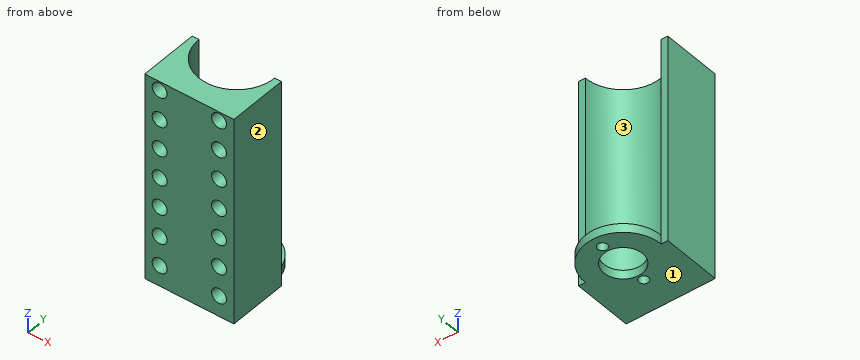
```python
from build123d import *

# Parameters (mm, degrees)
SKETCH1_R                = 12.75
SKETCH1_R_2              = 6.5
BOSS_EXTRUDE1_DEPTH      = 3
BOSS_EXTRUDE2_DEPTH      = 67
BOSS_EXTRUDE2_DEPTH_BACK = 3
SKETCH4_R                = 2.515
CUT_EXTRUDE1_DEPTH       = 6
LPATTERN1_COUNT          = 2
LPATTERN1_PITCH          = 20
LPATTERN1_COUNT_DIR2     = 7
LPATTERN1_PITCH_DIR2     = 10
SKETCH5_R                = 1.65
CUT_EXTRUDE2_DEPTH       = 75


with BuildPart() as part:
    # Sketch1 → Boss-Extrude1 (new body)
    with BuildSketch(Plane.XY):
        Circle(SKETCH1_R)
        Circle(SKETCH1_R_2, mode=Mode.SUBTRACT)
    extrude(amount=BOSS_EXTRUDE1_DEPTH)

    # Sketch2 → Boss-Extrude2 (add, two sides)
    with BuildSketch(Plane.XY.offset(3)) as boss_extrude2_sk:
        with BuildLine():
            Line((15, -20), (15, 0))
            Line((15, 0), (12.75, 0))
            ThreePointArc((12.75, 0), (0, -12.75), (-12.75, 0))
            Line((-12.75, 0), (-15, 0))
            Line((-15, 0), (-15, -20))
            Line((-15, -20), (15, -20))
        make_face()
    extrude(amount=BOSS_EXTRUDE2_DEPTH)
    extrude(boss_extrude2_sk.sketch, amount=-BOSS_EXTRUDE2_DEPTH_BACK)

    # Sketch4 → Cut-Extrude1 (cut)
    with BuildSketch(Plane.XZ.offset(20)):
        with Locations((-10, 67)):
            Circle(SKETCH4_R)
    cut_extrude1 = extrude(amount=-CUT_EXTRUDE1_DEPTH, mode=Mode.SUBTRACT)

    # LPattern1: Cut-Extrude1 2 × 7
    with Locations(*[(i * LPATTERN1_PITCH, 0, -j * LPATTERN1_PITCH_DIR2) for i in range(LPATTERN1_COUNT) for j in range(LPATTERN1_COUNT_DIR2) if (i, j) != (0, 0)]):
        add(cut_extrude1, mode=Mode.SUBTRACT)

    # Sketch5 → Cut-Extrude2 (cut)
    with BuildSketch(Plane(origin=(0, 0, 0), x_dir=(-1, 0, 0), z_dir=(0, 0, -1))):
        with Locations((0, 8.7)):
            Circle(SKETCH5_R)
        with Locations((0, -8.7)):
            Circle(SKETCH5_R)
    extrude(amount=-CUT_EXTRUDE2_DEPTH, mode=Mode.SUBTRACT)


solid = part.part
```
Geometry: final body of the model. Coordinates: model frame, mm. Face numbers are marked on the shaded views. Coordinates: 2 decimals unless noted, no trailing zeros. Write each loop counter-clockwise with the first axis right and the second up, starting at its lowest first coordinate (ties: lowest second). Pieces come first, ordered by that corner, then holes. Notation, with made-up numbers: M 45.25,4.5 L 50.25,4.5 A22 cw 50.25,20.5 Z; hole C -39,-25 d10. An arc over 180 degrees is marked long. Answer as CSV lines item,"result". Start each with the question number.
Q1. Mould query, pull axis X, two halves, no side actions, for the marked faces 1, 2 and 3. Classes: released by +X, released by -X, zero draft, split by the parting line, or undercut.
Q2. Line query: line 1 (Y direction, x = 0, z = 1.9); line 2 (X direction, y = -2.5, z = 40.5); line 3 (X direction, y = -11.5, z = 34). Output: solid intervals per line, ascending. Write a range as from..to.
Q3. Cut plane A-A on x = 0. Return the cut outline in (y, z).
Q4. Cut plane C-C on z = 37. Return the cut outline in (x, y) (3 decimals).
Q5. Cut plane B-B on y = 1. Return the cut outline in (x, z).
Q6. Cut plane D-D on x = 4.5. Return the cut outline in (y, z), then the cut area to 3 significant figures.
Q7. Pin query (flat end, axial travel): P1, Ø3, axis at x = 10, z = 37, coming from the +Y side; P2, Ø1.5, axis at x = -2, z = 33.5, coming from the +Y side; P3, Ø1.5, axis at x = 10.5, z = 16.5, coming from the -Y side; P4, Ø6.5, axis at x = 10, z = 17, coming from the -Y side. Return the tip coordinate at first contact, or that it passes through.
Findings below:
1,face 1,"zero draft"
1,face 2,"released by +X"
1,face 3,"undercut"
2,line 1,"y = -20..-10.35, -7.05..-6.5, 6.5..7.05, 10.35..12.75"
2,line 2,"x = -15..-12.5, 12.5..15"
2,line 3,"x = -15..-5.51, 5.51..15"
3,outline,"M -20,0 L -10.35,0 L -10.35,3 L -12.75,3 L -12.75,70 L -20,70 Z; M -7.05,0 L -6.5,0 L -6.5,3 L -7.05,3 Z; M 6.5,0 L 7.05,0 L 7.05,3 L 6.5,3 Z; M 10.35,0 L 12.75,0 L 12.75,3 L 10.35,3 Z"
4,outline,"M -15,-20 L -12.515,-20 L -12.515,-14 L -7.485,-14 L -7.485,-20 L 7.485,-20 L 7.485,-14 L 12.515,-14 L 12.515,-20 L 15,-20 L 15,0 L 12.75,0 A12.75 cw -12.75,0 L -15,0 Z"
5,outline,"M -12.71,0 L -6.42,0 L -6.42,3 L -12.71,3 Z; M 6.42,0 L 12.71,0 L 12.71,3 L 6.42,3 Z"
6,outline,"M -20,0 L -4.69,0 L -4.69,3 L -11.93,3 L -11.93,70 L -20,70 Z; M 4.69,0 L 11.93,0 L 11.93,3 L 4.69,3 Z"
6,area,"608 mm2"
7,P1,"stops at y = -5.51"
7,P2,"stops at y = -12.45"
7,P3,"stops at y = -14"
7,P4,"stops at y = -20"
